Geometry: final body of the model. Coordinates: model frame, mm. A direction names the side the tool comes from. Coordinates: 2 decimals unless noted, no trailing zeros. Order: outer loops, then holes, each group sorted by start corner. A loop starts at its lowest first (then second) coordinate and runs counter-clockwise, first axis right, second up. Notation, with made-up numbers: M -26.5,63.25 L -2.5,63.25 A20 cw -2.5,82.25 Z; hole C -3.75,32.25 d5. An arc over 180 degrees is marked long. One line per question, with ' | ' between items.
from build123d import *

# Parameters (mm, degrees)
BOSS_EXTRUDE1_DEPTH = 4
BOSS_EXTRUDE2_DEPTH = 24.6
BOSS_EXTRUDE3_DEPTH = 12.3
BOSS_EXTRUDE4_DEPTH = 12.3
BOSS_EXTRUDE5_DEPTH = 12.3
BOSS_EXTRUDE6_DEPTH = 3
CHAMFER1_SIZE       = 4
CHAMFER4_SIZE       = 2
CHAMFER5_SIZE       = 1
BOSS_EXTRUDE7_DEPTH = 3
CHAMFER8_SIZE       = 3
CHAMFER7_SIZE       = 1
CUT_EXTRUDE1_REACH  = 48.53
CUT_EXTRUDE2_REACH  = 50.101
CUT_EXTRUDE3_REACH  = 49.91
CUT_EXTRUDE4_REACH  = 49.91


with BuildPart() as part:
    # Sketch1 → Boss-Extrude1 (new body)
    with BuildSketch(Plane.XY):
        Polygon((-8.7625, 27.356), (-8.7625, 18.256), (0.832623943, -4.7625), (2.5, -8.7625), (10.5, -8.7625), (12.39611144, -6.261946641), (12.39611144, 11.881414246), (26.153799919, 11.881414246), (30.9875, 18.256), (30.9875, 27.356), align=None)
    extrude(amount=BOSS_EXTRUDE1_DEPTH)

    # Sketch1<5> → Boss-Extrude2 (add)
    with BuildSketch(Plane.XY):
        Polygon((2.5, -5.094), (2.5, -8.7625), (5.5, -8.7625), (5.5, -0.594), (2.5, -0.594), align=None)
    extrude(amount=-BOSS_EXTRUDE2_DEPTH)

    # Sketch2 → Boss-Extrude3 (add)
    with BuildSketch(Plane(origin=(0, 0, 0), x_dir=(-1, 0, 0), z_dir=(0, 0, -1))):
        Polygon((-27.45, 18.256), (-22.7, 18.256), (-22.7, 21.256), (-30.9875, 21.256), (-30.9875, 18.256), align=None)
    extrude(amount=BOSS_EXTRUDE3_DEPTH)

    # Sketch3 → Boss-Extrude4 (add)
    with BuildSketch(Plane(origin=(0, 0, 0), x_dir=(-1, 0, 0), z_dir=(0, 0, -1))):
        Polygon((0, 18.256), (4.75, 18.256), (8.7625, 18.256), (8.7625, 27.356), (0, 27.356), (0, 22.106), align=None)
    extrude(amount=BOSS_EXTRUDE4_DEPTH)

    # Sketch4 → Boss-Extrude5 (add)
    with BuildSketch(Plane(origin=(0, 0, -12.3), x_dir=(-1, 0, 0), z_dir=(0, 0, -1))):
        Polygon((4.1, 22.106), (4.1, 18.256), (7.1, 18.256), (7.1, 27.356), (0, 27.356), (0, 22.356), (3.85, 22.356), (4.1, 22.356), align=None)
    extrude(amount=BOSS_EXTRUDE5_DEPTH)

    # Sketch5 → Boss-Extrude6 (add)
    with BuildSketch(Plane.XZ.offset(8.7625)):
        Polygon((5.5, -15), (10.5, 0), (5.5, 0), align=None)
    extrude(amount=-BOSS_EXTRUDE6_DEPTH)

    # Chamfer1
    chamfer1_edges = [part.edges().sort_by_distance(p)[0] for p in [
        (4, -8.7625, -24.6),
    ]]
    chamfer(chamfer1_edges, length=CHAMFER1_SIZE)

    # Chamfer4
    # the kernel refuses this chamfer: 2 mm, written as the material it adds along each edge
    with BuildSketch(Plane(origin=(-7.1, 18.256, -12.3), x_dir=(-0.9996219169112973, 0, 0.027495876610566645), z_dir=(0, 1, 0))) as chamfer4_piece_1_section:
        Polygon((CHAMFER4_SIZE * 0.999621916911, -CHAMFER4_SIZE * 0.0274958766106), (-CHAMFER4_SIZE * 0.0274958766106, -CHAMFER4_SIZE * 0.999621916911), (0, 0), align=None)
    chamfer4_piece_1 = extrude(amount=9.1, mode=Mode.PRIVATE)
    chamfer4_piece_1 = split(chamfer4_piece_1, bisect_by=Plane(origin=(-8.7625, 22.806, -12.984491238), z_dir=(1, 0, 0)), keep=Keep.TOP, mode=Mode.PRIVATE)
    add(chamfer4_piece_1)

    # Chamfer5
    chamfer5_edges = [part.edges().sort_by_distance(p)[0] for p in [
        (-7.93125, 18.256, -13.46875),
        (-8.7625, 18.256, -6.31875),
        (-7.1, 22.806, -24.6),
        (-7.1, 18.256, -19.45),
    ]]
    chamfer(chamfer5_edges, length=CHAMFER5_SIZE)

    # Sketch6 → Boss-Extrude7 (add)
    with BuildSketch(Plane(origin=(30.9875, 0, 0), x_dir=(0, 0, -1), z_dir=(1, 0, 0))):
        Polygon((12.3, 21.256), (0, 27.356), (-0.5, 27.356), (-0.5, 20.756), (12.3, 20.756), align=None)
    extrude(amount=-BOSS_EXTRUDE7_DEPTH)

    # Chamfer8
    chamfer8_edges = [part.edges().sort_by_distance(p)[0] for p in [
        (12.39611144, 11.881414246, 2),
    ]]
    chamfer(chamfer8_edges, length=CHAMFER8_SIZE)

    # Chamfer7
    chamfer7_edges = [part.edges().sort_by_distance(p)[0] for p in [
        (11.44805572, -7.51222332, 4),
        (-3.13125, 4.74675, 0),
        (12.39611144, 1.309733803, 4),
        (13.89611144, 10.381414246, 4),
        (20.77495568, 11.881414246, 4),
        (28.57064996, 15.068707123, 4),
        (30.9875, 22.806, 4),
        (11.1125, 27.356, 4),
        (-8.7625, 22.806, 4),
        (-3.13125, 4.74675, 4),
        (6.5, -8.7625, 4),
    ]]
    chamfer(chamfer7_edges, length=CHAMFER7_SIZE)

    # Sketch7 → Cut-Extrude1 (cut, up to next)
    with BuildSketch(Plane.ZY.offset(-2.5), mode=Mode.PRIVATE) as cut_extrude1_sk1:
        with BuildLine():
            ThreePointArc((-18.7, -4.215214264), (-18.45, -4.244), (-18.2, -4.215214264))
            ThreePointArc((-18.2, -4.215214264), (-17.588315603, -3.827739717), (-17.35, -3.144))
            ThreePointArc((-17.35, -3.144), (-19.133739717, -2.282315603), (-18.7, -4.215214264))
        make_face()
    cut_extrude1_tool1 = extrude(cut_extrude1_sk1.sketch, amount=-CUT_EXTRUDE1_REACH, mode=Mode.PRIVATE) & part.part
    add(cut_extrude1_tool1.solids().sort_by_distance((2.5, -3.144, -18.45))[0], mode=Mode.SUBTRACT)

    # Sketch8 → Cut-Extrude2 (cut, up to next)
    with BuildSketch(Plane(origin=(0, 0, 0), x_dir=(0, 0, -1), z_dir=(1, 0, 0)), mode=Mode.PRIVATE) as cut_extrude2_sk1:
        with BuildLine():
            ThreePointArc((18.7, 26.227214264), (18.45, 26.256), (18.2, 26.227214264))
            ThreePointArc((18.2, 26.227214264), (17.766260283, 24.294315603), (19.55, 25.156))
            ThreePointArc((19.55, 25.156), (19.311684397, 25.839739717), (18.7, 26.227214264))
        make_face()
    cut_extrude2_tool1 = extrude(cut_extrude2_sk1.sketch, amount=-CUT_EXTRUDE2_REACH, mode=Mode.PRIVATE) & part.part
    add(cut_extrude2_tool1.solids().sort_by_distance((0, 25.156, -18.45))[0], mode=Mode.SUBTRACT)

    # Sketch9 → Cut-Extrude3 (cut, up to next)
    with BuildSketch(Plane.XZ.offset(-18.256), mode=Mode.PRIVATE) as cut_extrude3_sk1:
        with BuildLine():
            ThreePointArc((-3.871214264, -5.9), (-3.9, -6.15), (-3.871214264, -6.4))
            ThreePointArc((-3.871214264, -6.4), (-2.67417411, -7.24277987), (-1.7, -6.15))
            ThreePointArc((-1.7, -6.15), (-2.67417411, -5.05722013), (-3.871214264, -5.9))
        make_face()
    cut_extrude3_tool1 = extrude(cut_extrude3_sk1.sketch, amount=-CUT_EXTRUDE3_REACH, mode=Mode.PRIVATE) & part.part
    add(cut_extrude3_tool1.solids().sort_by_distance((-2.8, 18.256, -6.15))[0], mode=Mode.SUBTRACT)

    # Sketch10 → Cut-Extrude4 (cut, up to next)
    with BuildSketch(Plane.XZ.offset(-18.256), mode=Mode.PRIVATE) as cut_extrude4_sk1:
        with BuildLine():
            ThreePointArc((26.6, -6.15), (26.59277987, -6.02417411), (26.571214264, -5.9))
            ThreePointArc((26.571214264, -5.9), (24.4, -6.15), (26.571214264, -6.4))
            ThreePointArc((26.571214264, -6.4), (26.59277987, -6.27582589), (26.6, -6.15))
        make_face()
    cut_extrude4_tool1 = extrude(cut_extrude4_sk1.sketch, amount=-CUT_EXTRUDE4_REACH, mode=Mode.PRIVATE) & part.part
    add(cut_extrude4_tool1.solids().sort_by_distance((25.5, 18.256, -6.15))[0], mode=Mode.SUBTRACT)


solid = part.part
1. Section A-A, the plane x = -3. Output: boundary loops of the cut face in (y, z).
Response values:
outline: M 4.43,1 L 7.03,0 L 18.26,0 L 18.26,-5.07 L 27.36,-5.07 L 27.36,3 L 26.36,4 L 7.03,4 L 4.43,3 Z; M 18.26,-12.3 L 22.36,-12.3 L 22.36,-24.6 L 27.36,-24.6 L 27.36,-7.23 L 18.26,-7.23 Z; hole C 25.16,-18.45 d2.2
2. Section C-C, the plane y = 0.5. Output: boundary loops of the cut face in (x, z), and give its area (3 significant figures).
Response values:
outline: M -1.36,1 L -0.28,0 L 12.4,0 L 12.4,3 L 11.4,4 L -0.28,4 L -1.36,3 Z | area: 53.4 mm^2
3. Pin query (flat end, axial travel): P1, Ø2.5, axis at x = 7, z = -8.5, coming from the +Y side; P2, Ø4, axis at y = -1.5, z = -8.5, coming from the +X side; P3, Ø2.5, axis at x = 28.5, z = -5, coming from the -Y side; P4, Ø6, axis at x = 17.5, y = -3, coming from the -Z side. Return the tip coordinate at first contact, or that it passes through.
Response values:
P1: stops at y = -5.76 | P2: stops at x = 5.5 | P3: stops at y = 18.26 | P4: passes through
4. Section B-B, the plane z = -8. Output: boundary loops of the cut face in (x, y), and give its area (3 significant figures).
Response values:
outline: M -8.76,19.26 L -7.76,18.26 L 0,18.26 L 0,27.36 L -8.76,27.36 Z; M 2.5,-8.76 L 7.83,-8.76 L 7.83,-5.76 L 5.5,-5.76 L 5.5,-0.59 L 2.5,-0.59 Z; M 22.7,18.26 L 30.99,18.26 L 30.99,23.39 L 27.99,23.39 L 27.99,21.26 L 22.7,21.26 Z | area: 142 mm^2
5. Access query for faces 1 (the face through (20.49, 12.39, 3.51)), 2 (the face through (27, 20, -12.3)), 3 (the face through (7, -5.762, -6)), 4 (the face through (30.988, 22, -3)). Directions: +Z, -Z, +X, -X, +Y, -Y. A direction counts if a zero-diameter tool reaches every point of the face in a straight line with its end or side. Return the directions, or none.
Response values:
face 1: +Z, +X, -Y | face 2: -Z, +X, +Y, -Y | face 3: -Z, +X, +Y | face 4: +Z, -Z, +X, +Y, -Y
6. Section D-D, the plane x = 16. Output: boundary loops of the cut face in (y, z).
Response values:
outline: M 11.88,0 L 27.36,0 L 27.36,3 L 26.36,4 L 12.88,4 L 11.88,3 Z
7. Draft query along X for faces 5 (the face through (-7.1, 23, -19)), 6 (the face through (29.51, 24.26, -6.24)), 7 (the face through (11.03, -7.22, 3.51)), 8 (the face through (27.988, 23, -3)). Return one class per face: pulls with the +X half, pulls with the -X half, needs draft (parallel to the pull), parting line crosses it, or undercut.
Response values:
face 5: pulls with the -X half | face 6: needs draft | face 7: pulls with the +X half | face 8: undercut
8. Material intervals for line 1 (X direction, y = 19.5, z = -6.15); line 2 (X direction, y = 25, z = -2.5); line 3 (Y direction, x = -4.25, z = -18.45), sorted ascending. Write a range as [from, to].
Response values:
line 1: x = [-8.76, -3.9], [-1.7, 0], [22.7, 24.4], [26.6, 30.99] | line 2: x = [-8.76, 0], [27.99, 30.99] | line 3: y = [18.26, 24.06], [26.26, 27.36]
